from build123d import *

# Parameters (mm, degrees)
F_20_0_20_DURCHMESSER_BOHRUNG1_D = 20


with BuildPart() as part:
    # Skizze1 → Rotation1 (revolve)
    with BuildSketch(Plane(origin=(0, 0, 0), x_dir=(0, 0, -1), z_dir=(1, 0, 0)), mode=Mode.PRIVATE) as rotation1_sk:
        with BuildLine():
            Line((177.8, 0), (177.8, 8.537744837))
            ThreePointArc((177.8, 8.537744837), (171.896273488, 29.053926256), (155.991, 43.294360308))
            ThreePointArc((155.991, 43.294360308), (80.012631482, 69.959635546), (0, 79))
            Line((0, 79), (0, 76))
            ThreePointArc((0, 76), (79.343256428, 67.035266035), (154.686, 40.593068951))
            ThreePointArc((154.686, 40.593068951), (169.355112336, 27.459404384), (174.8, 8.537744837))
            Line((174.8, 8.537744837), (174.8, 0))
            Line((174.8, 0), (177.8, 0))
        make_face()
    revolve(rotation1_sk.sketch.rotate(Axis((0, 44.907564577, 0), (0, -1, 0)), 180), axis=Axis((0, 44.907564577, 0), (0, -1, 0)))  # turned: the seam where the file's is

    # Ø20.0 (20) Durchmesser Bohrung1 (through all)
    with Locations(Plane(origin=(86.602540378, 64.774737749, 50), x_dir=(0.969804385, -0.243884101, 0), z_dir=(0.241501786, 0.960331115, 0.139431121))):
        with Locations((0, 0)):
            Hole(F_20_0_20_DURCHMESSER_BOHRUNG1_D / 2)


solid = part.part
The model under review builds one solid part; all positions refer to its coordinate system, in mm. Round coordinates to 2 decimals unless told otherwise and drop trailing zeros. Order: outer loops, then holes, each group sorted by start corner. A loop starts at its lowest first (then second) coordinate and runs counter-clockwise, first axis right, second up. Notation, with made-up numbers: (-3.75, 9) -> (26.25, 9) arc R25 ccw to (26.25, 28) -> close; hole circle Ø4 at (3.5, 59). An arc over 180 degrees is marked (long way). Use CSV: the item, a comma, the result in double quotes. Start each with the question number.
(1) Mouldability with a two-part tool opening along X and no side actions: class faces 1 (the face through (118, 0, -131)), 2 (the face through (-120.166, 4.329, -131.046)), 3 (the face through (93.691, 60.421, 55.794)) as pulls with the +X half, pulls with the -X half, needs draft (parallel to the pull), parting line crosses it, or undercut.
(2) Consider section B-B on z = 0. Write out the cut boundary in (x, y).
(3) Consider section C-C on y = 29. Write out the cut boundary in (x, z).
(4) Consider section A-A on x = 0. Write out the cut boundary in (y, z), and give its area (3 significant figures).
(5) Insertion check: pin 1 (6 mm diameter, centred on y = 18.5, z = -68.5, fed in from +X); pin 2 (5 mm diameter, centred on x = -100, z = 24.5, fed in from +Y); pin 3 (4 mm diameter, centred on y = 22, z = 70.5, fed in from +X). Each pin has a flat end and moves straight along its axis. Give the tip position at first contact, or say it passes through.
(6) Wall thickness on probe 1 along X at (y, z) = (5, 0); probe 2 along Z at (x, y) = (-29, 26); probe 3 along X at (y, z) = (16, 34): over which ranges is each line inside the solid? List them lowest first. Write a range as from..to.
Responses:
1,face 1,"needs draft"
1,face 2,"parting line crosses it"
1,face 3,"undercut"
2,outline,"(-177.8, 0) -> (-174.8, 0) -> (-174.8, 8.54) arc R35.6 cw to (-154.69, 40.59) arc R355.6 cw to (154.69, 40.59) arc R35.6 cw to (174.8, 8.54) -> (174.8, 0) -> (177.8, 0) -> (177.8, 8.54) arc R38.6 ccw to (155.99, 43.29) arc R358.6 ccw to (-155.99, 43.29) arc R38.6 ccw to (-177.8, 8.54) -> close"
3,outline,"circle Ø343.86 at (0, 0); hole circle Ø336.66 at (0, 0)"
4,outline,"(0, -177.8) -> (8.54, -177.8) arc R38.6 ccw to (43.29, -155.99) arc R358.6 ccw to (43.29, 155.99) arc R38.6 ccw to (8.54, 177.8) -> (0, 177.8) -> (0, 174.8) -> (8.54, 174.8) arc R35.6 cw to (40.59, 154.69) arc R355.6 cw to (40.59, -154.69) arc R35.6 cw to (8.54, -174.8) -> (0, -174.8) -> close"
4,area,"1,260 mm²"
5,pin 1,"x = 164.12"
5,pin 2,"y = 64.64"
5,pin 3,"x = 161.74"
6,probe 1,"-177.8..-174.8, 174.8..177.8"
6,probe 2,"-171.19..-167.73, 167.73..171.19"
6,probe 3,"-173.78..-170.66, 170.66..173.78"
